```python
from build123d import *

# Parameters (mm, degrees)
F0_W     = 150
F0_H     = 125
F1_DEPTH = 48
F2_R     = 1.75
F2_W     = 9
F2_H     = 16
F3_DEPTH = 2
F4_R     = 1.75
F5_DEPTH = 2
F6_SIZE  = 2
F7_R     = 4


with BuildPart() as f1:
    # F0 (on Top) → F1 (new body)
    with BuildSketch(Plane.XY):
        Polygon((75, 89.5), (75, 64.5), (-75, 64.5), (-75, 89.5), (-77, 89.5), (-77, 64.5), (-77, -64.5), (77, -64.5), (77, 64.5), (77, 89.5), align=None)
        Rectangle(F0_W, F0_H, mode=Mode.SUBTRACT)
    extrude(amount=F1_DEPTH)

    # F2 (on face) → F3 (cut)
    with BuildSketch(Plane.XZ.offset(64.5)):
        with Locations((-65, 34.7)):
            Circle(F2_R)
        with Locations((-52, 34.7)):
            Circle(F2_R)
        with Locations((-65, 13.3)):
            Circle(F2_R)
        with Locations((-52, 13.3)):
            Circle(F2_R)
        with Locations((52, 34.7)):
            Circle(F2_R)
        with Locations((65, 34.7)):
            Circle(F2_R)
        with Locations((52, 13.3)):
            Circle(F2_R)
        with Locations((65, 13.3)):
            Circle(F2_R)
        with Locations((-35, 24)):
            Rectangle(F2_W, F2_H)
        with Locations((35, 24)):
            Rectangle(F2_W, F2_H)
    extrude(amount=-F3_DEPTH, mode=Mode.SUBTRACT)

    # F4 (on face) → F5 (cut)
    with BuildSketch(Plane.XZ.offset(-62.5)):
        with Locations((-44.25, 24)):
            Circle(F4_R)
        with Locations((44.25, 24)):
            Circle(F4_R)
    extrude(amount=-F5_DEPTH, mode=Mode.SUBTRACT)

    # F6
    f6_edges = [f1.edges().sort_by_distance(p)[0] for p in [
        (-75, 62.5, 24),
        (-75, -62.5, 24),
        (75, -62.5, 24),
        (75, 62.5, 24),
        (75, 64.5, 24),
        (-75, 64.5, 24),
    ]]
    chamfer(f6_edges, length=F6_SIZE)

    # F7
    f7_edges = [f1.edges().sort_by_distance(p)[0] for p in [
        (-39.5, -63.5, 16),
        (-30.5, -63.5, 16),
        (-30.5, -63.5, 32),
        (-39.5, -63.5, 32),
        (30.5, -63.5, 16),
        (39.5, -63.5, 16),
        (39.5, -63.5, 32),
        (30.5, -63.5, 32),
    ]]
    fillet(f7_edges, radius=F7_R)


solid = f1.part
```
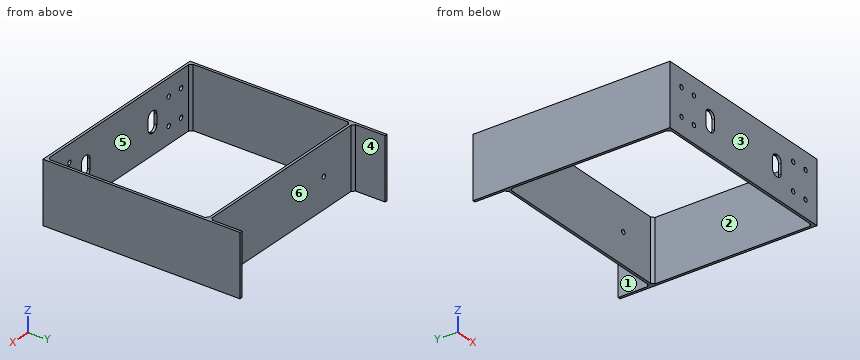
Verification items for the finished model (mm, model axes). Face numbers are marked on the shaded views. A direction names the side the tool comes from. Round coordinates to 2 decimals unless told otherwise and drop trailing zeros. Write each loop counter-clockwise with the first axis right and the second up, starting at its lowest first coordinate (ties: lowest second). Pieces come first, ordered by that corner, then holes. Notation, with made-up numbers: (-32, 88) - (-7, 88) arc R25 ccw to (-7, 101) - close; hole circle Ø4 at (51.25, -9). An arc over 180 degrees is marked (long way). Answer as a JSON object with one key per item and string values. Group by question number.
Q1. Mould release check, pull along Y, two halves, no side actions. Record for the marked faces 4, 5 and 6: released by +Y, released by -Y, zero draft, split by the parting line, or undercut.
Q2. Section check C-C, the plane x = 15.5. Enter the section's corners in (y, z).
Q3. Section check A-A, the plane z = 39. Enter the section's corners in (x, y), plus the area to 3 significant figures.
Q4. Section check B-B, the plane y = -49. Enter the section's corners in (x, z).
Q5. Thickness scan on line 1 (Z direction, x = -65, y = -64); line 2 (X direction, y = -63, z = 13); line 3 (X direction, y = 41, z = 37). Record the ranges inside material, lowest first.
Q6. Tool access check on the marked faces 1, 2 and 3. Record the directions out of +Z, -Z, +X, -X, +Y, -Y that give a thin tool (end or side, any length) a straight path to the whole face; none if there is none.
Q7. Go/stop test with flat-tipped pins: pin 1 Ø6 at (x, z) = (3, 13) entering from +Y; pin 2 Ø3 at (x, z) = (44.25, 24) entering from +Y. Record where each tip stops, or that it passes through.
Found:
{
 "1": {"face 4": "zero draft", "face 5": "undercut", "face 6": "released by +Y"},
 "2": {"outline": "(-64.5, 0) - (-62.5, 0) - (-62.5, 48) - (-64.5, 48) - close; (62.5, 0) - (64.5, 0) - (64.5, 48) - (62.5, 48) - close"},
 "3": {"outline": "(-77, -64.5) - (77, -64.5) - (77, 89.5) - (75, 89.5) - (75, 66.5) - (73, 64.5) - (-73, 64.5) - (-75, 66.5) - (-75, 89.5) - (-77, 89.5) - close; hole (-75, -60.5) - (-73, -62.5) - (73, -62.5) - (75, -60.5) - (75, 60.5) - (73, 62.5) - (-73, 62.5) - (-75, 60.5) - close", "area": "1,230 mm^2"},
 "4": {"outline": "(-77, 0) - (-75, 0) - (-75, 48) - (-77, 48) - close; (75, 0) - (77, 0) - (77, 48) - (75, 48) - close"},
 "5": {"line 1": "z = 0 to 11.55, 15.05 to 32.95, 36.45 to 48", "line 2": "x = -77 to -66.72, -63.28 to -53.72, -50.28 to 50.28, 53.72 to 63.28, 66.72 to 77", "line 3": "x = -77 to -75, 75 to 77"},
 "6": {"face 1": "+Z, -Z, +Y", "face 2": "+Z, -Z", "face 3": "+Z, -Z, +X, -X, -Y"},
 "7": {"pin 1": "stops at y = 64.5", "pin 2": "stops at y = -62.5"}
}
